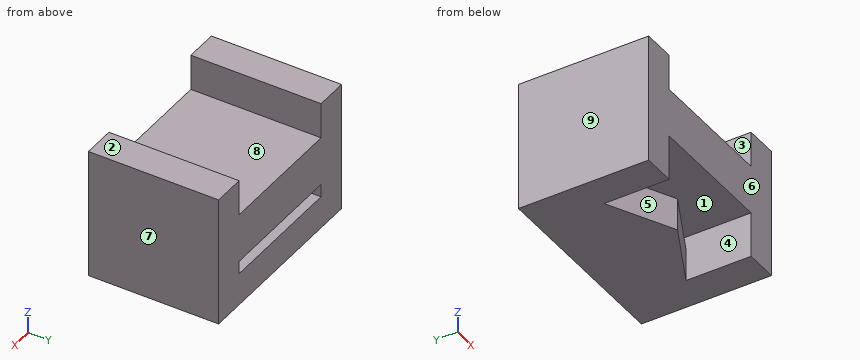
```python
from build123d import *

# Parameters (mm, degrees)
F0_W     = 20
F0_H     = 10
F1_DEPTH = 10
F2_DEPTH = 40
F3_START = 14
F3_DEPTH = 15


with BuildPart() as f1:
    # F0 (on Top) → F1 (new body)
    with BuildSketch(Plane.XY):
        with Locations((20, 35)):
            Rectangle(F0_W, F0_H)
        with Locations((40, 35)):
            Rectangle(F0_W, F0_H)
        with Locations((40, 25)):
            Rectangle(F0_W, F0_H)
        with Locations((20, 25)):
            Rectangle(F0_W, F0_H)
        Polygon((10, 20), (30, 10), (30, 20), align=None)
        Polygon((30, 20), (30, 10), (50, 20), align=None)
    extrude(amount=F1_DEPTH)

    # F0 (on Top) → F2 (join)
    with BuildSketch(Plane.XY):
        Polygon((0, 40), (0, 0), (10, 0), (10, 10), (10, 20), (10, 30), (10, 40), align=None)
        Polygon((50, 10), (50, 0), (60, 0), (60, 40), (50, 40), (50, 30), (50, 20), align=None)
    extrude(amount=F2_DEPTH)

    # F0 (on Top) → F3 (join)
    with BuildSketch(Plane.XY.offset(F3_START)):
        with Locations((40, 35)):
            Rectangle(F0_W, F0_H)
        with Locations((20, 35)):
            Rectangle(F0_W, F0_H)
        with Locations((20, 25)):
            Rectangle(F0_W, F0_H)
        with Locations((40, 25)):
            Rectangle(F0_W, F0_H)
        Polygon((10, 20), (30, 10), (30, 20), align=None)
        Polygon((30, 20), (30, 10), (50, 20), align=None)
        with Locations((40, 5)):
            Rectangle(F0_W, F0_H)
        with Locations((20, 5)):
            Rectangle(F0_W, F0_H)
        Polygon((10, 20), (10, 10), (30, 10), align=None)
        Polygon((50, 20), (30, 10), (50, 10), align=None)
    extrude(amount=F3_DEPTH)


solid = f1.part
```
Model file for the job. Use its own axes, mm. Face numbers are marked on the shaded views. A direction names the side the tool comes from. Give positions to 0.01 mm unless a question says otherwise; leave off trailing zeros. Write each loop counter-clockwise with the first axis right and the second up, starting at its lowest first coordinate (ties: lowest second). Pieces come first, ordered by that corner, then holes. Notation, with made-up numbers: M 43.5,-2.5 L 67.5,-2.5 A25 ccw 67.5,24.5 Z; hole C 17,23.5 d5. An arc over 180 degrees is marked long. Use a Markdown table: item, result.
1) Cut at D-D (y = 27). List the corners of the cut face in (x, z).
Responses:
| item | result |
|---|---|
| outline | M 0,0 L 60,0 L 60,40 L 50,40 L 50,29 L 10,29 L 10,40 L 0,40 Z; hole M 10,10 L 50,10 L 50,14 L 10,14 Z |
2) Pull direction X, two halves, no side cores. Call the marked faces 6, 7, 8 and 9: +X half, -X half, draft (parallel to the pull), parting line (faces both ways), or undercut.
Responses:
| item | result |
|---|---|
| face 6 | draft |
| face 7 | +X half |
| face 8 | undercut |
| face 9 | -X half |
3) Tool access for the marked faces 1, 2, 3, 4 and 5: list every direction of +Z, -Z, +X, -X, +Y, -Y with a clear straight run to the whole face (end or side of a thin tool).
Responses:
| item | result |
|---|---|
| face 1 | +Y, -Y |
| face 2 | +Z, +X, -X, +Y, -Y |
| face 3 | +Z, +Y, -Y |
| face 4 | -Y |
| face 5 | -Z, -Y |
4) Drill centre lines: line 1 (Z direction, x = 49, y = 36); line 2 (X direction, y = 8, z = 7); line 3 (X direction, y = 10.5, z = 2). Where is each one in solid material? Low to high. Write a range as from..to.
Responses:
| item | result |
|---|---|
| line 1 | z = 0..10, 14..29 |
| line 2 | x = 0..10, 50..60 |
| line 3 | x = 0..10, 29..31, 50..60 |
5) Cut at B-B (x = 24). List the corners of the cut face in (y, z).
Responses:
| item | result |
|---|---|
| outline | M 0,14 L 40,14 L 40,29 L 0,29 Z; M 13,0 L 40,0 L 40,10 L 13,10 Z |
6) Cut at C-C (y = 14). List the corners of the cut face in (x, z).
Responses:
| item | result |
|---|---|
| outline | M 0,0 L 10,0 L 10,14 L 50,14 L 50,0 L 60,0 L 60,40 L 50,40 L 50,29 L 10,29 L 10,40 L 0,40 Z; M 22,0 L 38,0 L 38,10 L 22,10 Z |
7) Pin check, flat tips, straight feed: pin 1 (24 mm diameter, centred on x = 25, y = 19, fed in from +Z); pin 2 (1.5 mm diameter, centred on x = 42.5, z = 9, fed in from -Y) (3 decimals). Stop position of each tip, or through.
Responses:
| item | result |
|---|---|
| pin 1 | stops at z = 29 |
| pin 2 | stops at y = 15.875 |
8) Cut at A-A (z = 30). List the corners of the cut face in (x, y).
Responses:
| item | result |
|---|---|
| outline | M 0,0 L 10,0 L 10,40 L 0,40 Z; M 50,0 L 60,0 L 60,40 L 50,40 Z |
